from build123d import *

# Parameters (mm, degrees)
F0_W     = 63.5
F0_H     = 38.1
F1_DEPTH = 25.4
F2_R     = 6.35
F2_R_2   = 3.175
F3_DEPTH = 50.8


with BuildPart() as f1:
    # F0 (on Top) → F1 (new body)
    with BuildSketch(Plane.XY):
        with Locations((-25.567356, -14.020799)):
            Rectangle(F0_W, F0_H)
    extrude(amount=F1_DEPTH)

    # F2 (on face) → F3 (join)
    with BuildSketch(Plane.XY.offset(25.4)):
        with Locations((-25.567356, -14.020799)):
            Circle(F2_R)
        with Locations((-25.567356, -14.020799)):
            Circle(F2_R_2, mode=Mode.SUBTRACT)
    extrude(amount=F3_DEPTH)


solid = f1.part
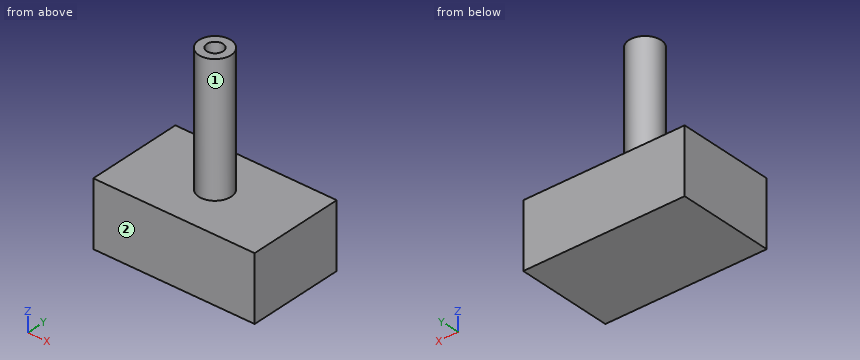
Geometry check sheet. Reference: the model listing, model coordinates, mm. Face numbers are marked on the shaded views. A direction names the side the tool comes from. Give positions to 0.01 mm unless a question says otherwise; leave off trailing zeros. Order: outer loops, then holes, each group sorted by start corner. A loop starts at its lowest first (then second) coordinate and runs counter-clockwise, first axis right, second up. Notation, with made-up numbers: (15, 45) - (37, 45) arc R21 ccw to (37, 78) - close; hole circle Ø1 at (79.25, 45.5). An arc over 180 degrees is marked (long way). Answer as a JSON object with one key per item and string values.
(1) Tool access check on the marked faces 1 and 2. Record the directions out of +Z, -Z, +X, -X, +Y, -Y that give a thin tool (end or side, any length) a straight path to the whole face; none if there is none.
Report:
{"face 1": "+Z", "face 2": "+Z, -Z, +X, -X, -Y"}
(2) Depth check by flat-ended pin: pin 1 Ø6 at (y, z) = (-4, 36) entering from +X; pin 2 Ø8 at (x, z) = (-26.5, 31) entering from +Y; pin 3 Ø11.5 at (x, y) = (-35, -23.5) entering from +Z; pin 4 Ø12 at (x, z) = (-14, 56) entering from +Y. Enter the tip coordinate at first touch or a pass-through.
Report:
{"pin 1": "through", "pin 2": "y = -7.67", "pin 3": "z = 25.4", "pin 4": "y = -10.97"}
(3) Material ranges on line 1 (X direction, y = -15, z = 54.5); line 2 (Z direction, x = -50, y = -0.5); line 3 (X direction, y = -18, z = 39), recorded low to high.
Report:
{"line 1": "-31.84 to -28.59, -22.55 to -19.29", "line 2": "0 to 25.4", "line 3": "-30.52 to -20.62"}
(4) Cross-section at A-A (y = -13). Record the cut outline in (x, z), then the cut area to 3 significant figures.
Report:
{"outline": "(-57.32, 0) - (6.18, 0) - (6.18, 25.4) - (-19.3, 25.4) - (-19.3, 76.2) - (-22.56, 76.2) - (-22.56, 25.4) - (-28.57, 25.4) - (-28.57, 76.2) - (-31.83, 76.2) - (-31.83, 25.4) - (-57.32, 25.4) - close", "area": "1,940 mm^2"}
(5) Cross-section at C-C (z = 64.5). Record the cut outline in (x, y) (3 decimals).
Report:
{"outline": "circle Ø12.7 at (-25.567, -14.021); hole circle Ø6.35 at (-25.567, -14.021)"}
(6) Cross-section at D-D (y = -2). Record the cut outline in (x, z).
Report:
{"outline": "(-57.32, 0) - (6.18, 0) - (6.18, 25.4) - (-57.32, 25.4) - close"}
(7) Cross-section at B-B (x = -25). Record the cut outline in (y, z), then the cut area to 3 significant figures.
Report:
{"outline": "(-33.07, 0) - (5.03, 0) - (5.03, 25.4) - (-7.7, 25.4) - (-7.7, 76.2) - (-10.9, 76.2) - (-10.9, 25.4) - (-17.14, 25.4) - (-17.14, 76.2) - (-20.35, 76.2) - (-20.35, 25.4) - (-33.07, 25.4) - close", "area": "1,290 mm^2"}
